```python
from build123d import *

# Parameters (mm, degrees)
SKETCH_1_R      = 6.5
SKETCH_1_R_2    = 4
EXTRUDE_1_DEPTH = 5
FILLET_1_R      = 0.5


with BuildPart() as part:
    # 草图1 → 凸台-拉伸1 (new body)
    with BuildSketch(Plane.XY):
        Circle(SKETCH_1_R)
        Circle(SKETCH_1_R_2, mode=Mode.SUBTRACT)
    extrude(amount=EXTRUDE_1_DEPTH)

    # 圆角1
    fillet_1_edges = [part.edges().sort_by_distance(p)[0] for p in [
        (-6.5, 0, 0),
        (-6.5, 0, 5),
        (-4, 0, 5),
    ]]
    fillet(fillet_1_edges, radius=FILLET_1_R)


solid = part.part
```
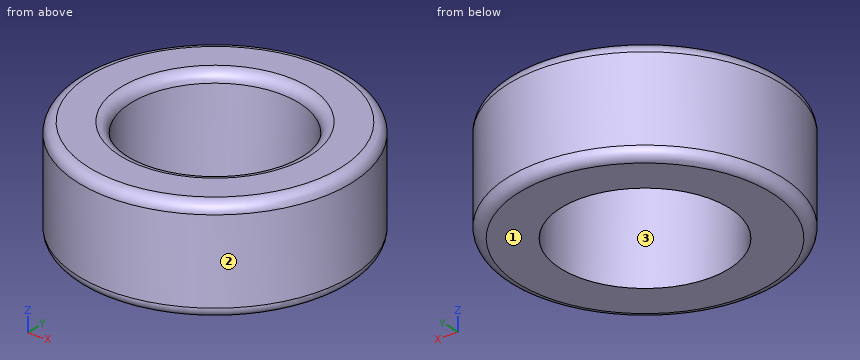
Geometry: final body of the model. Coordinates: model frame, mm. Face numbers are marked on the shaded views. Coordinates: 2 decimals unless noted, no trailing zeros. Order: outer loops, then holes, each group sorted by start corner. A loop starts at its lowest first (then second) coordinate and runs counter-clockwise, first axis right, second up. Notation, with made-up numbers: (-15, 38.25) -> (27, 38.25) arc R26 cw to (27, 66.25) -> close; hole circle Ø5 at (45.5, 85.5). An arc over 180 degrees is marked (long way). Write each question's results on one line, items separated by ' | '. Start each with the question number.
1) Cut plane C-C, the plane z = 1.15. Output: boundary loops of the cut face in (x, y).
2) First-contact query: pin 1 (1.5 mm diameter, centred on x = -4, z = 2, fed in from +Y); pin 2 (1 mm diameter, centred on x = 3, z = 2, fed in from +Y). Flat tips, straight axial feed; report the tip coordinate or a pass-through.
3) Material intervals for line 1 along Y through (x, z) = (0, 3.35); line 2 along X through (y, z) = (-2.5, 1.6); line 3 along X through (y, z) = (-2.75, 1.4), sorted ascending.
4) Cut plane A-A, the plane y = 0. Output: boundary loops of the cut face in (x, z).
5) Mould query, pull axis Y, two halves, no side actions, for the marked faces 1, 2 and 3. Classes: released by +Y, released by -Y, zero draft, split by the parting line, or undercut.
Checks:
1) outline: circle Ø13 at (0, 0); hole circle Ø8 at (0, 0)
2) pin 1: y = 5.63 | pin 2: y = 6
3) line 1: -6.5 to -4, 4 to 6.5 | line 2: -6 to -3.12, 3.12 to 6 | line 3: -5.89 to -2.9, 2.9 to 5.89
4) outline: (-6.5, 0.5) arc R0.5 ccw to (-6, 0) -> (-4, 0) -> (-4, 4.5) arc R0.5 ccw to (-4.5, 5) -> (-6, 5) arc R0.5 ccw to (-6.5, 4.5) -> close; (4, 0) -> (6, 0) arc R0.5 ccw to (6.5, 0.5) -> (6.5, 4.5) arc R0.5 ccw to (6, 5) -> (4.5, 5) arc R0.5 ccw to (4, 4.5) -> close
5) face 1: zero draft | face 2: split by the parting line | face 3: undercut
